from build123d import *

# Parameters (mm, degrees)
BOSS_EXTRUDE1_DEPTH   = 9.525
FILLET1_R             = 2.54
SKETCH5_R             = 1.5875
CUT_EXTRUDE1_DEPTH    = 39.578536455
F_8_32_TAPPED_HOLE1_D = 3.4544


with BuildPart() as part:
    # Sketch1 → Boss-Extrude1 (new body)
    with BuildSketch(Plane.XY):
        with BuildLine():
            Line((3.175, 6.985), (3.175, 0))
            ThreePointArc((3.175, 0), (0, -3.175), (-3.175, 0))
            Line((-3.175, 0), (-3.175, 13.335))
            Line((-3.175, 13.335), (31.75, 13.335))
            ThreePointArc((31.75, 13.335), (34.925, 10.16), (31.75, 6.985))
            Line((31.75, 6.985), (3.175, 6.985))
        make_face()
    extrude(amount=BOSS_EXTRUDE1_DEPTH)

    # Fillet1
    fillet1_edges = [part.edges().sort_by_distance(p)[0] for p in [
        (3.175, 6.985, 4.7625),
        (-3.175, 13.335, 4.7625),
    ]]
    fillet(fillet1_edges, radius=FILLET1_R)

    # Sketch5 → Cut-Extrude1 (cut, through all)
    with BuildSketch(Plane.XY.offset(9.525)):
        with Locations((0, 10.16)):
            Circle(SKETCH5_R)
    extrude(amount=-CUT_EXTRUDE1_DEPTH, mode=Mode.SUBTRACT)

    # #8-32 Tapped Hole1 (through all)
    with Locations(Plane.XY.offset(9.525)):
        with Locations((31.75, 10.16)):
            Hole(F_8_32_TAPPED_HOLE1_D / 2)


solid = part.part
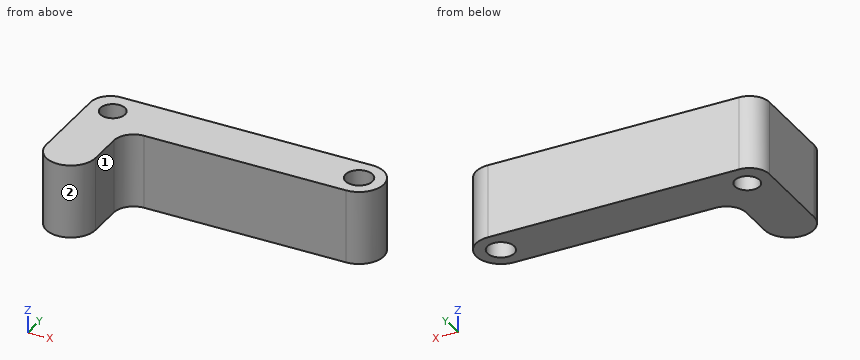
Can you work these out from the model? Positions are in its coordinate system, mm. Face numbers are marked on the shaded views. A direction names the side the tool comes from. Give positions to 0.01 mm unless a question says otherwise; leave off trailing zeros. Order: outer loops, then holes, each group sorted by start corner. A loop starts at its lowest first (then second) coordinate and runs counter-clockwise, first axis right, second up. Notation, with made-up numbers: M -20,-3 L 33,-3 A20 cw 33,9 Z; hole C -23.5,-34 d7. An arc over 180 degrees is marked long. One line per item, written item: value.
Item 1: For the marked faces 1 and 2, which set-ups out of +Z, -Z, +X, -X, +Y, -Y let a thin tool reach every point of the face, with its end or its side?
Verdict:
face 1: +Z, -Z, +X, -Y
face 2: +Z, -Z, -Y
Item 2: If we section it at D-D on y = 3: Write out the boundary of the cut face in (x, z) (3 decimals), and give its area (3 significant figures).
Verdict:
outline: M -3.175,0 L 3.175,0 L 3.175,9.525 L -3.175,9.525 Z
area: 60.5 mm2
Item 3: If we section it at B-B on x = 0: Write out the boundary of the cut face in (y, z) (1 decimal), and give its area (3 significant figures).
Verdict:
outline: M -3.2,0 L 8.6,0 L 8.6,9.5 L -3.2,9.5 Z; M 11.7,0 L 13.3,0 L 13.3,9.5 L 11.7,9.5 Z
area: 127 mm2
Item 4: If we section it at C-C on z = 8.75: State how many separate pieces and enclosed holes the cut face has, and give its area (3 significant figures).
Verdict:
separate pieces: 1
enclosed holes: 2
area: 281 mm2
Item 5: If we section it at A-A on y = 10.16: Write out the boundary of the cut face in (x, z) (1 decimal).
Verdict:
outline: M -3.2,0 L -1.6,0 L -1.6,9.5 L -3.2,9.5 Z; M 1.6,0 L 30,0 L 30,9.5 L 1.6,9.5 Z; M 33.5,0 L 34.9,0 L 34.9,9.5 L 33.5,9.5 Z
Item 6: Please list where these lines run through material, in increasing order: line 1 (X direction, y = 11.5, z = 6.5); line 2 (Y direction, x = 31.75, z = 5) (3 decimals); line 3 (Y direction, x = 0, z = 6.75) (1 decimal).
Verdict:
line 1: -3.08 to -0.85, 0.85 to 30.66, 32.84 to 34.63
line 2: 6.985 to 8.433, 11.887 to 13.335
line 3: -3.2 to 8.6, 11.7 to 13.3
Item 7: For pin 1 (4 mm diameter, centred on x = 31.75, y = 10.16, fed in from -Z); pin 2 (5 mm diameter, centred on y = 1.5, z = 2.5, fed in from +X) (3 decimals), each with a flat end and sliding along its axis, tell me the tip position at first contact or that it passes through.
Verdict:
pin 1: z = 0
pin 2: x = 3.175
